Drawing for the job (mm, zero at the part's lowest x, y, z). A direction names the side the tool comes from. Round coordinates to 2 decimals unless told otherwise and drop trailing zeros. Loops run counter-clockwise (first coordinate to the right, second up) from the corner with the lowest first, then second, coordinate; pieces in that order, holes last.
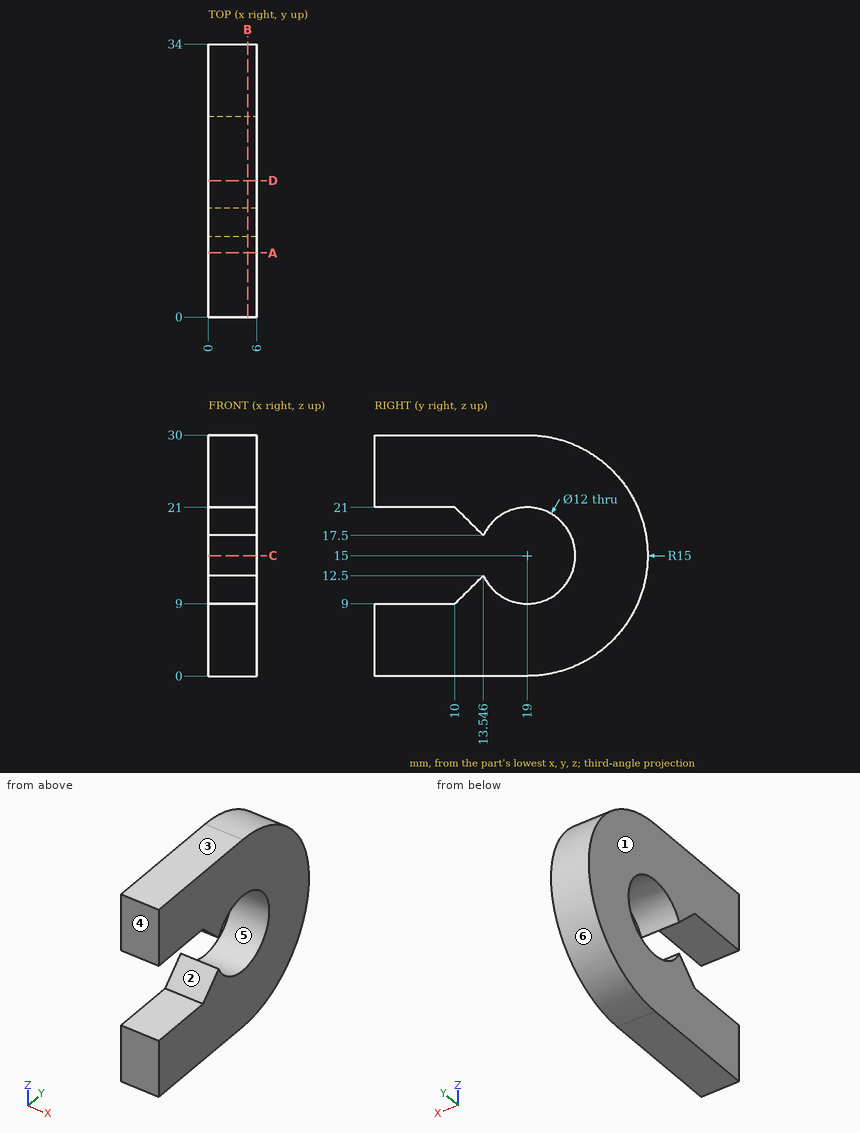
Q1. Slice it at B-B on x = 4.9. Give the cut face in (y, z) (1 decimal), plus the area to 3 significant figures.
Q2. Slice it at A-A on y = 8. Give the cut face in (x, z).
Q3. Tool access for the marked faces 1 and 2: list every direction of +Z, -Z, +X, -X, +Y, -Y with a clear straight run to the whole face (end or side of a thin tool).
Q4. Pull direction Y, two halves, no side cores. Call the marked faces 3, 4, 5 and 6: pulls with the +Y half, pulls with the -Y half, needs draft (parallel to the pull), parting line crosses it, or undercut.
Q5. Slice it at C-C on z = 15. Give the cut face in (x, y), plus the area to 3 significant figures.
Q6. Probe line 1 (Z direction, x = 1.85, y = 19); line 2 (Y direction, x = 4.35, z = 15); line 3 (Y direction, x = 1.7, z = 9.5) (1 decimal). List the from-to ranges inside material, lowest first.
Q7. Slice it at D-D on y = 17. Give the cut face in (x, z).
Reply:
1. outline: (0, 0) - (19, 0) arc R15 ccw to (19, 30) - (0, 30) - (0, 21) - (10, 21) - (13.5, 17.5) arc R6 cw (long way) to (13.5, 12.5) - (10, 9) - (0, 9) - close
1. area: 662 mm2
2. outline: (0, 0) - (6, 0) - (6, 9) - (0, 9) - close; (0, 21) - (6, 21) - (6, 30) - (0, 30) - close
3. face 1: +Z, -Z, -X, +Y, -Y
3. face 2: +X, -X, -Y
4. face 3: needs draft
4. face 4: pulls with the -Y half
4. face 5: undercut
4. face 6: pulls with the +Y half
5. outline: (0, 25) - (6, 25) - (6, 34) - (0, 34) - close
5. area: 54.0 mm2
6. line 1: z = 0 to 9, 21 to 30
6. line 2: y = 25 to 34
6. line 3: y = 10.5 to 16.6, 21.4 to 33
7. outline: (0, 0) - (6, 0) - (6, 9.34) - (0, 9.34) - close; (0, 20.66) - (6, 20.66) - (6, 30) - (0, 30) - close
